Design review of the part built by this model. Coordinates are the model's own, in mm. A direction names the side the tool comes from. Coordinates: 2 decimals unless noted, no trailing zeros. Loops run counter-clockwise (first coordinate to the right, second up) from the corner with the lowest first, then second, coordinate; pieces in that order, holes last.
Q1. Add section D-D on y = -7. Give the boundary of the cut face in (x, z) (3 decimals), and give its area (3 significant figures).
Q2. Machinability: for faces 1 (the face through (3.131, 6.452, -19.706)), 2 (the face through (3, -6, -6.825)), 3 (the face through (3, 0, -15)), which of the approach directions +Z, -Z, +X, -X, +Y, -Y give a long, thin tool a straight path to every point of the face, cutting with its end or side? Answer none if there is none.
Q3. For P1, Ø0.6, axis at x = 4, y = 10.5, coming from the +Z side; P2, Ø2.5, axis at y = 2.43, z = -10, coming from the +X side; P3, Ø3, axis at x = 2, y = -4.5, coming from the -Z side (3 decimals); P4, Ø3, axis at x = 2.5, y = 28, coming from the +Z side (3 decimals), all flat-tipped, find the tip position at first contact; note any pin that passes through.
Q4. Wall thickness on probe 1 along Y at (x, z) = (1.5, -10); probe 2 along Z at (x, y) = (4.5, -3) (3 decimals); probe 3 along Y at (x, z) = (1.5, -5): over which ranges is each line inside the solid? List them lowest first.
Q5. Draft analysis for pull direction Y (two halves, no side actions). For faces 4 (the face through (3, 29, -13.175)), 5 (the face through (3.131, 0.724, -19.236)), 6 (the face through (3.131, 12.367, -14.863)), state which applies: released by +Y, released by -Y, zero draft, split by the parting line, or undercut.
Q6. Add section B-B on z = -2. Give the boundary of the cut face in (x, y).
Q7. Add section C-C on x = 5.25. Give the number of separate pieces and of enclosed holes in the cut face, and give its area (3 significant figures).
Q8. Add section A-A on z = -10. Give the boundary of the cut face in (x, y), and give its area (3 significant figures).
```python
from build123d import *

# Parameters (mm, degrees)
SKETCH1_R           = 1.49987
BOSS_EXTRUDE1_DEPTH = 6.35
FILLET1_R           = 2.54


with BuildPart() as part:
    # Sketch1 → Boss-Extrude1 (new body)
    with BuildSketch(Plane(origin=(0, 0, 0), x_dir=(0, 0, -1), z_dir=(1, 0, 0))):
        Polygon((0, 0), (6.825, 0), (6.825, -12.7), (13.175, -12.7), (13.175, 0), (20, 0), (20, 6.629574014), (14.471500996, 10.288392178), (14.471500996, 12.377602622), (20, 16.036420786), (20, 22.6659948), (13.175, 22.6659948), (13.175, 35.3659948), (6.825, 35.3659948), (6.825, 22.6659948), (0, 22.6659948), (0, 16.036420786), (5.528499004, 12.377602622), (5.528499004, 10.288392178), (0, 6.629574014), align=None)
        with Locations((10, 19.9520048)):
            Circle(SKETCH1_R, mode=Mode.SUBTRACT)
        with Locations((10, 2.4260048)):
            Circle(SKETCH1_R, mode=Mode.SUBTRACT)
    extrude(amount=BOSS_EXTRUDE1_DEPTH)

    # Fillet1
    # the kernel refuses this fillet: 2.54 mm, written as the material it adds along each edge
    with BuildSketch(Plane(origin=(0, 12.377602622, -14.471500996), x_dir=(0, -1, 0), z_dir=(1, 0, 0)), Plane(origin=(0, 10.288392178, -14.471500996), x_dir=(0, -0.5518934032294348, -0.8339146667806201), z_dir=(1, 0, 0)), Plane(origin=(0, 12.377602622, -5.528499004), x_dir=(0, 0.5518934032294354, 0.8339146667806197), z_dir=(1, 0, 0))) as fillet1_piece_1:
        with BuildLine():
            CenterArc((FILLET1_R * 0.537353058558, FILLET1_R), FILLET1_R, 213.497005554, 56.502994446)
            Line((-FILLET1_R * 0.296561608223, FILLET1_R * 0.448106596771), (0, 0))
            Line((0, 0), (FILLET1_R * 0.537353058558, 0))
        make_face()
    extrude(amount=6.35)
    # the kernel refuses this fillet: 2.54 mm, written as the material it takes off along each edge
    with BuildSketch(Plane(origin=(-3.412191922, 16.036420786, -20), x_dir=(0, -0.5518934032294348, 0.8339146667806201), z_dir=(1, 0, 0)), Plane(origin=(-3.412191922, 6.629574014, -20), x_dir=(0, -1, 0), z_dir=(1, 0, 0)), Plane(origin=(-3.412191922, 16.036420786, 0), x_dir=(0, 1, 0), z_dir=(1, 0, 0))) as fillet1_2_piece_1:
        with BuildLine():
            CenterArc((FILLET1_R * 0.537353058558, -FILLET1_R), FILLET1_R, 90, 56.502994446)
            Line((-FILLET1_R * 0.296561608223, -FILLET1_R * 0.448106596771), (0, 0))
            Line((0, 0), (FILLET1_R * 0.537353058558, 0))
        make_face()
    extrude(amount=13.174383844, mode=Mode.SUBTRACT)
    with BuildSketch(Plane(origin=(-6.35, 0, -20), x_dir=(0, 0, 1), z_dir=(1, 0, 0)), Plane(origin=(-6.35, 22.6659948, 0), x_dir=(0, 0, -1), z_dir=(1, 0, 0)), Plane(origin=(-6.35, 22.6659948, -20), x_dir=(0, -1, 0), z_dir=(1, 0, 0))) as fillet1_2_piece_2:
        with BuildLine():
            CenterArc((FILLET1_R, -FILLET1_R), FILLET1_R, 90, 90)
            Line((0, -FILLET1_R), (0, 0))
            Line((0, 0), (FILLET1_R, 0))
        make_face()
    extrude(amount=19.05, mode=Mode.SUBTRACT)
    with BuildSketch(Plane(origin=(-6.35, 0, 0), x_dir=(0, 0, -1), z_dir=(1, 0, 0))) as fillet1_2_piece_3:
        with BuildLine():
            CenterArc((FILLET1_R, FILLET1_R), FILLET1_R, 180, 90)
            Line((0, FILLET1_R), (0, 0))
            Line((0, 0), (FILLET1_R, 0))
        make_face()
    extrude(amount=19.05, mode=Mode.SUBTRACT)
    with BuildSketch(Plane(origin=(-3.412191922, 6.629574014, 0), x_dir=(0, -1, 0), z_dir=(1, 0, 0))) as fillet1_2_piece_4:
        with BuildLine():
            CenterArc((FILLET1_R * 0.537353058558, FILLET1_R), FILLET1_R, 213.497005554, 56.502994446)
            Line((-FILLET1_R * 0.296561608223, FILLET1_R * 0.448106596771), (0, 0))
            Line((0, 0), (FILLET1_R * 0.537353058558, 0))
        make_face()
    extrude(amount=13.174383844, mode=Mode.SUBTRACT)


solid = part.part
```
Entries:
1. outline: (0, -13.175) - (6.35, -13.175) - (6.35, -6.825) - (0, -6.825) - close
1. area: 40.3 mm2
2. face 1: -Z, +X, -X
2. face 2: +Z, +X, -X, -Y
2. face 3: -Z, +X, -X, -Y
3. P1: stops at z = -5.39
3. P2: passes through
3. P3: stops at z = -13.175
3. P4: stops at z = -6.825
4. probe 1: y = -12.7 to 0.93, 3.93 to 18.45, 21.45 to 35.37
4. probe 2: z = -13.175 to -6.825
4. probe 3: y = 0 to 9.94, 12.56 to 22.67
5. face 4: zero draft
5. face 5: released by -Y
5. face 6: undercut
6. outline: (0, 0.06) - (6.35, 0.06) - (6.35, 7.95) - (0, 7.95) - close; (0, 14.71) - (6.35, 14.71) - (6.35, 22.61) - (0, 22.61) - close
7. separate pieces: 1
7. enclosed holes: 2
7. area: 531 mm2
8. outline: (0, -12.7) - (6.35, -12.7) - (6.35, 0.93) - (0, 0.93) - close; (0, 3.93) - (6.35, 3.93) - (6.35, 18.45) - (0, 18.45) - close; (0, 21.45) - (6.35, 21.45) - (6.35, 35.37) - (0, 35.37) - close
8. area: 267 mm2
